from build123d import *

# Parameters (mm, degrees)
F0_W     = 1092.2
F0_H     = 1219.2
F1_DEPTH = 225.425
F2_W     = 152.4
F2_H     = 136.525
F3_DEPTH = 1092.2


with BuildPart() as f1:
    # F0 (on Top) → F1 (new body)
    with BuildSketch(Plane.XY):
        with Locations((0, -609.6)):
            Rectangle(F0_W, F0_H)
    extrude(amount=-F1_DEPTH)

    # F2 (on face) → F3 (cut, through all)
    with BuildSketch(Plane.YZ.offset(546.1)):
        with Locations((-1143, -157.1625)):
            Rectangle(F2_W, F2_H)
    extrude(amount=-F3_DEPTH, mode=Mode.SUBTRACT)


solid = f1.part
Design review of the part built by this model. Coordinates are the model's own, in mm. A direction names the side the tool comes from. Coordinates: 2 decimals unless noted, no trailing zeros. Write each loop counter-clockwise with the first axis right and the second up, starting at its lowest first coordinate (ties: lowest second). Pieces come first, ordered by that corner, then holes. Notation, with made-up numbers: (41.5, 16) - (46.5, 16) arc R27 cw to (46.5, 49) - close; hole circle Ø8 at (53.5, 43). An arc over 180 degrees is marked (long way). One line per item, written item: value.
1) For faces 1 (the face through (8, -1066.8, -158)), 2 (the face through (546.1, -618, -111)), list the 3-axis set-ups (+Z, -Z, +X, -X, +Y, -Y) from which the entire face can be reached by the end or side of a thin tool; tool diameter is ignored.
Answer sheet:
face 1: -Z, +X, -X, -Y
face 2: +Z, -Z, +X, +Y, -Y
2) Mouldability with a two-part tool opening along Z and no side actions: class faces 3 (the face through (-8, 0, -111)), 4 (the face through (-8, -526, -225.425)), 5 (the face through (-8, -601, 0)) as +Z half, -Z half, draft (parallel to the pull), parting line (faces both ways), or undercut.
Answer sheet:
face 3: draft
face 4: -Z half
face 5: +Z half
3) To check wall thickness, follow probe 1 along Y at (x, z) = (-359, -118). State the ranges of the line that lie inside material, in increasing order.
Answer sheet:
probe 1: y = -1066.8 to 0
4) Add section B-B (z = -113.5). State the section outline as (x, y) points.
Answer sheet:
outline: (-546.1, -1066.8) - (546.1, -1066.8) - (546.1, 0) - (-546.1, 0) - close
5) Insertion check: pin 1 (3 mm diameter, centred on x = -413.5, z = -110.5, fed in from -Y). The pin has a flat end and moves straight along its axis. Give the tip position at first contact, or say it passes through.
Answer sheet:
pin 1: stops at y = -1066.8
6) Add section A-A (x = -260.5). State the section outline as (y, z) points (3 decimals), plus the area to 3 significant figures.
Answer sheet:
outline: (-1219.2, -88.9) - (-1066.8, -88.9) - (-1066.8, -225.425) - (0, -225.425) - (0, 0) - (-1219.2, 0) - close
area: 254,000 mm2
